Verification items for the finished model (mm, model axes). Round coordinates to 2 decimals unless told otherwise and drop trailing zeros. Write each loop counter-clockwise with the first axis right and the second up, starting at its lowest first coordinate (ties: lowest second). Pieces come first, ordered by that corner, then holes. Notation, with made-up numbers: M 78,-37 L 109,-37 A23 ccw 109,-7 Z; hole C -10,14 d1. An arc over 180 degrees is marked long. One line per item, written item: value. Start each with the question number.
Item 1: Section check C-C, the plane x = -2. Record the cut outline in (y, z).
Item 2: Section check A-A, the plane z = 0.6. State how many separate pieces and enclosed holes the cut face has, then the cut area to 3 significant figures.
Item 3: Gauge pin test, flat ends, axial feed: pin 1 (18 mm diameter, centred on x = 0, y = 0, fed in from +Z); pin 2 (1.5 mm diameter, centred on x = -7, z = 0.5, fed in from -Y); pin 3 (0.9 mm diameter, centred on y = -77.5, z = 1.5, fed in from +X); pin 4 (0.9 mm diameter, centred on y = -52, z = 2, fed in from -X). Record the tip position at first contact, or that the pin passes through.
Item 4: Thickness scan on probe 1 along X at (y, z) = (-37.5, 2.45); probe 2 along Y at (x, z) = (2.5, 0.8); probe 3 along Y at (x, z) = (-0.5, 1.3). Record the ranges inside material, lowest first. Write a range as from..to.
Item 5: Section check B-B, the plane y = 4. Record the cut outline in (x, z).
Item 6: Section check D-D, the plane x = 12.5. Record the cut outline in (y, z), then the cut area to 3 significant figures.
from build123d import *

# Parameters (mm, degrees)
F1_DEPTH = 3
F2_R     = 10
F3_DEPTH = 25
F4_R     = 7.49999
F6_DEPTH = 25


# Not quite as in the source:
# - a fillet or chamfer is up to 0.001 mm smaller than in the source, because OpenCascade refuses the exact size


with BuildPart() as f1:
    # F0 (on Top) → F1 (new body)
    with BuildSketch(Plane.XY):
        with BuildLine():
            Line((7.5, -16.9115345253), (7.5, 16.9115345253))
            ThreePointArc((7.5, 16.9115345253), (0, 18.5), (-7.5, 16.9115345253))
            Line((-7.5, 16.9115345253), (-7.5, -16.9115345253))
            ThreePointArc((-7.5, -16.9115345253), (0, -18.5), (7.5, -16.9115345253))
        make_face()
        with BuildLine():
            Line((-7.5, -16.9115345253), (-7.5, 16.9115345253))
            ThreePointArc((-7.5, 16.9115345253), (-18.5, 0), (-7.5, -16.9115345253))
        make_face()
        with BuildLine():
            ThreePointArc((7.5, -16.9115345253), (15.5080624193, -10.0871205009), (18.5, 0))
            ThreePointArc((18.5, 0), (15.5080624193, 10.0871205009), (7.5, 16.9115345253))
            Line((7.5, 16.9115345253), (7.5, -16.9115345253))
        make_face()
        with BuildLine():
            Line((7.5, -100), (7.5, -16.9115345253))
            ThreePointArc((7.5, -16.9115345253), (0, -18.5), (-7.5, -16.9115345253))
            Line((-7.5, -16.9115345253), (-7.5, -100))
            Line((-7.5, -100), (7.5, -100))
        make_face()
    extrude(amount=F1_DEPTH)

    # F2 (on face) → F3 (cut)
    with BuildSketch(Plane.XY.offset(3)):
        Circle(F2_R)
    extrude(amount=-F3_DEPTH, mode=Mode.SUBTRACT)

    # F4 (radius 7.5 in the source; OpenCascade refuses exactly that, so slightly less here)
    f4_edges = [f1.edges().sort_by_distance(p)[0] for p in [
        (7.5, -100, 1.5),
        (-7.5, -100, 1.5),
    ]]
    fillet(f4_edges, radius=F4_R)

    # F5 (on face) → F6 (cut)
    with BuildSketch(Plane.XY.offset(3)):
        with BuildLine():
            ThreePointArc((-3, -92.5), (0, -95.5), (3, -92.5))
            Line((3, -92.5), (3, -32.5))
            ThreePointArc((3, -32.5), (0, -29.5), (-3, -32.5))
            Line((-3, -32.5), (-3, -92.5))
        make_face()
    extrude(amount=-F6_DEPTH, mode=Mode.SUBTRACT)


solid = f1.part
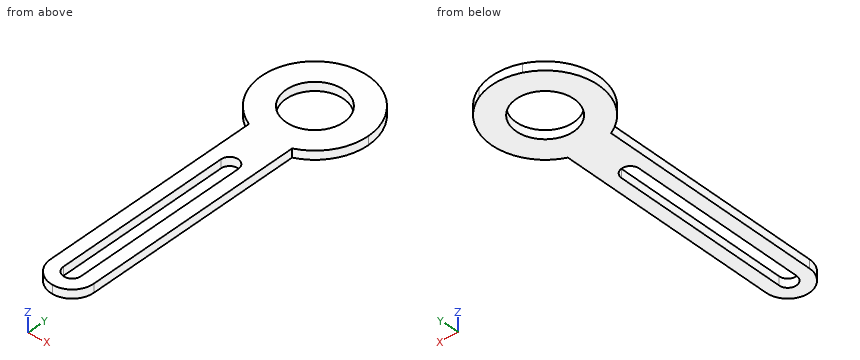
Response values:
1. outline: M -99.73,0 L -94.74,0 L -94.74,3 L -99.73,3 Z; M -30.26,0 L -9.8,0 L -9.8,3 L -30.26,3 Z; M 9.8,0 L 18.39,0 L 18.39,3 L 9.8,3 Z
2. separate pieces: 1
2. enclosed holes: 2
2. area: 1,580 mm2
3. pin 1: passes through
3. pin 2: stops at y = -96.65
3. pin 3: stops at x = 7.5
3. pin 4: stops at x = -7.5
4. probe 1: x = -7.5..-3, 3..7.5
4. probe 2: y = -99.57..-94.16, -30.84..-9.68, 9.68..18.33
4. probe 3: y = -99.98..-95.46, -29.54..-9.99, 9.99..18.49
5. outline: M -18.06,0 L -9.17,0 L -9.17,3 L -18.06,3 Z; M 9.17,0 L 18.06,0 L 18.06,3 L 9.17,3 Z
6. outline: M -13.64,0 L 13.64,0 L 13.64,3 L -13.64,3 Z
6. area: 81.8 mm2
